Can you work these out from the drawing? Everything is in mm from the part's minimum corner. Give positions to 0.01 mm unless a question says otherwise; leave off trailing zeros. Loops run counter-clockwise (first coordinate to the right, second up) from the corner with the lowest first, then second, coordinate; pieces in that order, holes last. Notation, with made-up numbers: (78, 20.5) -> (122, 20.5) arc R22 ccw to (122, 55.5) -> close; hole circle Ø5 at (19.5, 12.25). An arc over 180 degrees is marked (long way). Write item = value, one per line. Start each with the question number.
1) I want a section at A-A (y = 88.9). List the corners of the cut face in (x, z) for me.
2) I need wall thicknesses on probe 1 along Z at (x, y) = (71, 190); probe 2 along Z at (x, y) = (63, 241). Which ranges of each line are inside material? Lowest first, please. Write a range as from..to.
3) I want a section at B-B (x = 9). Count the separate pieces of the cut face and the enclosed holes in it, and give its area (3 significant figures).
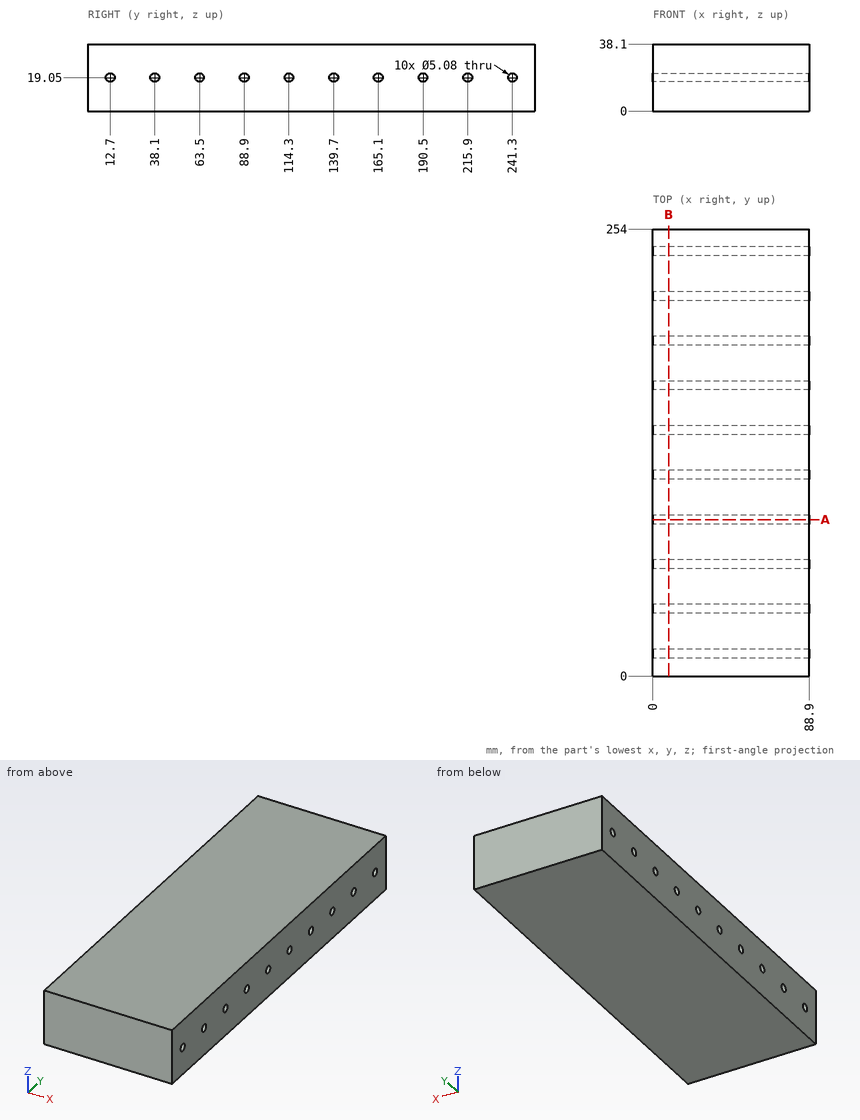
Answer list:
q1.outline = (0, 0) -> (88.9, 0) -> (88.9, 16.51) -> (0, 16.51) -> close; (0, 21.59) -> (88.9, 21.59) -> (88.9, 38.1) -> (0, 38.1) -> close
q2.probe_1 = 0..16.56, 21.54..38.1
q2.probe_2 = 0..16.53, 21.57..38.1
q3.separate_pieces = 1
q3.enclosed_holes = 10
q3.area = 9,470 mm^2
